Design review of the part built by this model. Coordinates are the model's own, in mm. A direction names the side the tool comes from. Round coordinates to 2 decimals unless told otherwise and drop trailing zeros. Order: outer loops, then holes, each group sorted by start corner. A loop starts at its lowest first (then second) coordinate and runs counter-clockwise, first axis right, second up.
from build123d import *

# Parameters (mm, degrees)
F0_W     = 50.8
F0_H     = 76.2
F1_DEPTH = 50.8
F2_W     = 25.4
F2_H     = 38.1
F3_DEPTH = 50.8
F4_W     = 38.1
F4_H     = 25.4
F5_DEPTH = 25.4
F6_W     = 38.1
F6_H     = 25.4
F7_DEPTH = 25.4


with BuildPart() as f1:
    # F0 (on Front) → F1 (new body)
    with BuildSketch(Plane.XZ):
        with Locations((-25.4, -38.1)):
            Rectangle(F0_W, F0_H)
    extrude(amount=-F1_DEPTH)

    # F2 (on face) → F3 (cut)
    with BuildSketch(Plane.XY):
        with Locations((-25.4, 31.75)):
            Rectangle(F2_W, F2_H)
    extrude(amount=-F3_DEPTH, mode=Mode.SUBTRACT)

    # F4 (on face) → F5 (cut)
    with BuildSketch(Plane(origin=(-50.8, 0, 0), x_dir=(0, -1, 0), z_dir=(-1, 0, 0))):
        with Locations((-31.75, -12.7)):
            Rectangle(F4_W, F4_H)
    extrude(amount=-F5_DEPTH, mode=Mode.SUBTRACT)

    # F6 (on face) → F7 (cut)
    with BuildSketch(Plane.YZ):
        with Locations((31.75, -12.7)):
            Rectangle(F6_W, F6_H)
    extrude(amount=-F7_DEPTH, mode=Mode.SUBTRACT)


solid = f1.part
1) The part is to be moulded in two halves that separate along X. For faces 4 (the face through (-26, 12.7, -20)), 5 (the face through (-26, 32, -50.8)), 6 (the face through (-50.8, 25, -47)), 7 (the face through (-6, 31, -25.4)), say which applies: released by +X, released by -X, zero draft, split by the parting line, or undercut.
Results:
face 4: undercut
face 5: undercut
face 6: released by -X
face 7: zero draft
2) Take a section at A-A on y = 28. Give the boundary of the cut face in (x, z), plus the area to 3 significant figures.
Results:
outline: (-50.8, -76.2) - (0, -76.2) - (0, -25.4) - (-12.7, -25.4) - (-12.7, -50.8) - (-38.1, -50.8) - (-38.1, -25.4) - (-50.8, -25.4) - close
area: 1,940 mm2
3) Clearance check with flat-ended pins moving along their axes: P1, Ø20.5, axis at x = -20.5, y = 39.5, coming from the +Z side; P2, Ø8, axis at x = -32, y = 23.5, coming from the +Z side. State where each tip first meets the part, or that it passes through.
Results:
P1: stops at z = -25.4
P2: stops at z = -50.8
4) For faces 1 (the face through (-12.7, 31, -38)), 2 (the face through (-45, 32, -25.4)), 3 (the face through (-26, 25, -76.2)), list the 3-axis set-ups (+Z, -Z, +X, -X, +Y, -Y) from which the entire face can be reached by the end or side of a thin tool; tool diameter is ignored.
Results:
face 1: +Z, +Y
face 2: +Z, +X, -X, +Y
face 3: -Z, +X, -X, +Y, -Y
5) Take a section at B-B on z = -43. Give the boundary of the cut face in (x, y), plus the area to 3 significant figures.
Results:
outline: (-50.8, 0) - (0, 0) - (0, 50.8) - (-12.7, 50.8) - (-12.7, 12.7) - (-38.1, 12.7) - (-38.1, 50.8) - (-50.8, 50.8) - close
area: 1,610 mm2
6) To check wall thickness, follow line 1 along X through (y, z) = (25, -39.5); line 2 along Y through (x, z) = (-22, -30); line 3 along Z through (x, y) = (-48, 16). State the ranges of each line that lie inside material, in increasing order.
Results:
line 1: x = -50.8 to -38.1, -12.7 to 0
line 2: y = 0 to 12.7
line 3: z = -76.2 to -25.4
7) Take a section at C-C on x = -40.5. Give the boundary of the cut face in (y, z).
Results:
outline: (0, -76.2) - (50.8, -76.2) - (50.8, -25.4) - (12.7, -25.4) - (12.7, 0) - (0, 0) - close
8) Take a section at D-D on x = -27. Give the boundary of the cut face in (y, z).
Results:
outline: (0, -76.2) - (50.8, -76.2) - (50.8, -50.8) - (12.7, -50.8) - (12.7, 0) - (0, 0) - close
